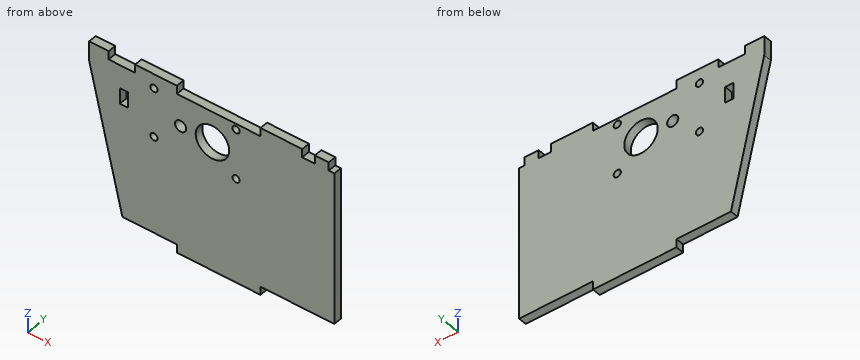
from build123d import *

# Parameters (mm, degrees)
SKETCH1_R           = 2
SKETCH1_R_2         = 6
SKETCH1_R_3         = 1.3
SKETCH1_W           = 3
SKETCH1_H           = 5.696795919
BOSS_EXTRUDE1_DEPTH = 3


with BuildPart() as part:
    # Sketch1 → Boss-Extrude1 (new body)
    with BuildSketch(Plane(origin=(0, 0, 0), x_dir=(1, 0, 0), z_dir=(0, 1, 0))):
        Polygon((-95.740581995, 27.853387647), (-80.740581995, 27.853387647), (-80.740581995, 30.853387647), (-50.740581995, 30.853387647), (-50.740581995, 27.853387647), (-35.740581995, 27.853387647), (-26.240581995, 27.853387647), (-24.240581995, 27.853387647), (-24.240581995, -27.146612353), (-26.240581995, -27.146612353), (-26.240581995, -30.146612353), (-31.240581995, -30.146612353), (-31.240581995, -27.146612353), (-35.740581995, -27.146612353), (-35.740581995, -30.146612353), (-50.740581995, -30.146612353), (-50.740581995, -27.146612353), (-80.740581995, -27.146612353), (-80.740581995, -30.146612353), (-95.740581995, -30.146612353), (-95.740581995, -27.146612353), (-105.240581995, -27.146612353), (-105.240581995, -30.146612353), (-112.240581995, -30.146612353), (-112.240581995, -27.146612353), (-112.240581995, -23.146612353), (-100.290581995, 27.853387647), align=None)
        with Locations(Location((-79.383372271, -16.032348928, 0), (0, 0, 270))):
            Circle(SKETCH1_R, mode=Mode.SUBTRACT)
        with Locations(Location((-67.983372271, -16.032348928, 0), (0, 0, 270))):
            Circle(SKETCH1_R_2, mode=Mode.SUBTRACT)
        with Locations(Location((-59.483372271, -25.032348928, 0), (0, 0, 270))):
            Circle(SKETCH1_R_3, mode=Mode.SUBTRACT)
        with Locations(Location((-59.483372271, -7.032348928, 0), (0, 0, 270))):
            Circle(SKETCH1_R_3, mode=Mode.SUBTRACT)
        with Locations(Location((-88.98337227, -7.23234893, 0), (0, 0, 270))):
            Circle(SKETCH1_R_3, mode=Mode.SUBTRACT)
        with Locations(Location((-88.98337227, -24.93234893, 0), (0, 0, 270))):
            Circle(SKETCH1_R_3, mode=Mode.SUBTRACT)
        with Locations((-99.720235087, -15.880746888)):
            Rectangle(SKETCH1_W, SKETCH1_H, mode=Mode.SUBTRACT)
    extrude(amount=BOSS_EXTRUDE1_DEPTH)


solid = part.part
Input: part model. Units: mm. Frame: model coordinates. Give positions to 0.01 mm unless a question says otherwise; leave off trailing zeros. Loops run counter-clockwise (first coordinate to the right, second up) from the corner with the lowest first, then second, coordinate; pieces in that order, holes last. Notation, with made-up numbers: (8.5, -36.5) - (53.5, -36.5) arc R24 ccw to (53.5, -1.5) - close; hole circle Ø7 at (51, 7.5). An arc over 180 degrees is marked (long way). Use CSV: the item, a comma, the result in double quotes. Start each with the question number.
Item 1: Section D-D on x = -33. Return loops of the section in (y, z).
Item 2: Section C-C on y = 0.6. State how many separate pieces and enclosed holes the cut face has, then the cut area to 3 significant figures.
Item 3: Line query: line 1 (X direction, y = 2.15, z = 25); line 2 (Z direction, x = -74.5, y = 2.7); line 3 (Z direction, x = -84, y = 2.3). Output: solid intervals per line, ascending.
Item 4: Section B-B on z = 20. Return loops of the section in (x, y), then the cut area to 3 significant figures.
Item 5: Contact query for flat-ended pins moving along their axis: P1, Ø0.9, axis at y = 1.5, z = 28.5, coming from the +X side; P2, Ø1.5, axis at x = -87, y = 1, coming from the -Z side; P3, Ø0.9, axis at x = -65, y = 1.5, coming from the +Z side. Output: stop coordinate, or through.
Item 6: Section A-A on x = -72. Return loops of the section in (y, z), then the cut area to 3 significant figures.
Ans:
1,outline,"(0, -27.85) - (3, -27.85) - (3, 27.15) - (0, 27.15) - close"
2,separate pieces,"1"
2,enclosed holes,"7"
2,area,"4,590 mm2"
3,line 1,"x = -112.24 to -90.28, -87.69 to -60.78, -58.18 to -24.24"
3,line 2,"z = -30.85 to 27.15"
3,line 3,"z = -27.85 to 30.15"
4,outline,"(-111.5, 0) - (-72.48, 0) - (-72.48, 3) - (-111.5, 3) - close; (-63.48, 0) - (-24.24, 0) - (-24.24, 3) - (-63.48, 3) - close"
4,area,"235 mm2"
5,P1,"stops at x = -26.24"
5,P2,"stops at z = -27.85"
5,P3,"stops at z = 27.15"
6,outline,"(0, -30.85) - (3, -30.85) - (3, 11.58) - (0, 11.58) - close; (0, 20.49) - (3, 20.49) - (3, 27.15) - (0, 27.15) - close"
6,area,"147 mm2"
